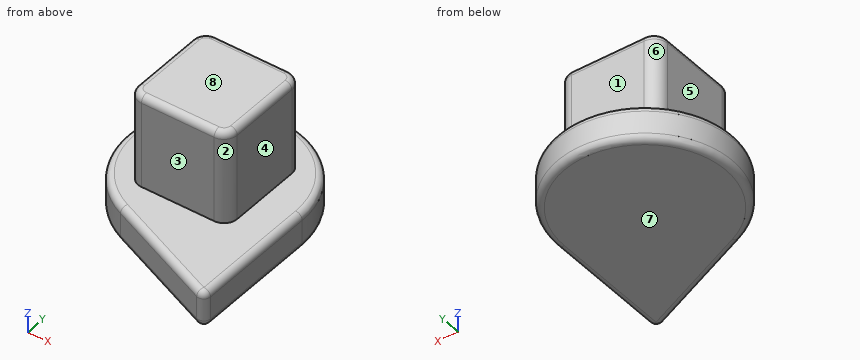
Autodesk Inventor part; units mm, degrees
ref_plane "YZ Plane" through (0, 0, 0) normal (1, 0, 0) x (0, 1, 0)
ref_plane "XZ Plane" through (0, 0, 0) normal (0, 1, 0) x (-1, 0, 0)
ref_plane "XY Plane" through (0, 0, 0) normal (0, 0, 1) x (1, 0, 0)
ref_plane "Work Plane1" through (0, 0, 0) normal (0, 0, 1) x (1, 0, 0)
sketch "Sketch1" plane through (0, 0, 0) normal (0, 0, 1) x (1, 0, 0)
  line L0 (57, -9.5) -> (57, -71.5)
  line L1 (71, -71.5) -> (71, -9.5)
  line L2 (71, -40.5) -> (57, -40.5) construction
  circle A0 centre (64, -40.5) radius 7 construction
  circle A1 centre (64, -40.5) radius 6.6
  line L3 (70.6, -40.5) -> (70.6, -50.5)
  line L4 (70.6, -50.5) -> (61.4052, -46.5685)
  point P0 (0, 0)
  dimension "d0" = 0.4
  dimension "d1" = 10
extrude "Extrusion1" add sketch "Sketch1" along normal blind 2.7
sketch "Sketch2" plane through (0, 0, 2.7) normal (0, 0, 1) x (1, 0, 0)
  line L0 (61.4052, -46.5685) -> (70.6, -50.5)
  line L1 (70.6, -50.5) -> (70.6, -40.5)
  arc A0 (70.6, -40.5) -> (61.4052, -46.5685) centre (64, -40.5) ccw
  line L2 (58.5, -71.5) -> (58.5, -11) construction
  line L3 (69.5, -11) -> (69.5, -71.5) construction
  circle A1 centre (64, -40.5) radius 5.5 construction
  line L4 (60.2523, -36.7523) -> (67.7477, -36.7523)
  line L5 (67.7477, -36.7523) -> (67.7477, -44.2477)
  line L6 (67.7477, -44.2477) -> (60.2523, -44.2477)
  line L7 (60.2523, -44.2477) -> (60.2523, -36.7523)
  line L8 (60.0396, -36.6836) -> (67.9604, -44.3164) construction
  line L9 (67.7477, -36.7523) -> (60.2523, -44.2477) construction
  circle A2 centre (64, -40.5) radius 5.3
  point P0 (0, 0)
  dimension "d11" = 7.4953
  dimension "d12" = 7.4953
  dimension "d14" = 0.2
extrude "Extrusion2" add sketch "Sketch2" along normal blind 7 contours L4 L5 L6 L7
fillet "Fillet1" radius 1 4 edges at (60.2523, -44.2477, 6.2) (60.2523, -36.7523, 6.2) (67.7477, -36.7523, 6.2) (67.7477, -44.2477, 6.2)
fillet "Fillet2" radius 0.5 8 edges at (67.4548, -43.9548, 9.7) (67.7477, -40.5, 9.7) (67.4548, -37.0452, 9.7) (64, -36.7523, 9.7) (60.5452, -37.0452, 9.7) (60.2523, -40.5, 9.7) (60.5452, -43.9548, 9.7) (64, -44.2477, 9.7)
fillet "Fillet3" radius 0.5 7 edges at (60.3644, -34.9916, 2.7) (70.6, -45.5, 2.7) (66.0026, -48.5343, 2.7) (60.3644, -34.9916, 0) (70.6, -45.5, 0) (66.0026, -48.5343, 0) (70.6, -50.5, 1.35)
equation "\"d12\" = d11"
properties part number "Arm"
Source: CAD feature listing. Evaluate the final solid. Frame: model axes, mm. Face numbers are marked on the shaded views. A direction names the side the tool comes from. Give positions to 0.01 mm unless a question says otherwise; leave off trailing zeros. Write each loop counter-clockwise with the first axis right and the second up, starting at its lowest first coordinate (ties: lowest second). Pieces come first, ordered by that corner, then holes. Notation, with made-up numbers: (24.5, 38.25) - (67.5, 38.25) arc R21 cw to (67.5, 62.25) - close; hole circle Ø8 at (-39, -19). An arc over 180 degrees is marked (long way). Write item = value, one per line. Start each with the question number.
Q1. Material intervals for probe 1 along Z at (x, y) = (59.75, -37.25); probe 2 along Y at (x, z) = (62.75, 4); probe 3 along X at (y, z) = (-43.25, 6.5), sorted ascending.
Q2. Reachability of the marked faces 1, 2, 3, 4 and 5 from +Z, -Z, +X, -X, +Y, -Y: full face, straight path, thin tool, end or side. Return the list, or none.
Q3. Pin query (flat end, axial travel): pin 1 Ø1.6 at (y, z) = (-41.5, 7.5) entering from -X; pin 2 Ø4 at (y, z) = (-42.5, 6.5) entering from +X; pin 3 Ø1.6 at (x, z) = (64, 5) entering from +Y. Return the tip coordinate at first contact, or that it passes through.
Q4. Cut plane A-A, the plane z = 9. Return loops of the section in (x, y), then the cut area to 3 significant figures.
Q5. Cut plane C-C, the plane z = 2.5. Return loops of the section in (x, y).
Q6. Draft query along Z for the marked faces 6, 7 and 8. Return one class per face: +Z half, -Z half, draft (parallel to the pull), parting line (faces both ways), or undercut.
Q7. Cut plane B-B, the plane z = 1. Return loops of the section in (x, y), then the cut area to 3 significant figures.
Computed values:
q1.probe_1 = 0 to 2.7
q1.probe_2 = -44.25 to -36.75
q1.probe_3 = 60.25 to 67.75
q2.face_1 = +Z, +X, -X, +Y
q2.face_2 = +Z, +X, -Y
q2.face_3 = +Z, +X, -X, -Y
q2.face_4 = +Z, +X, +Y, -Y
q2.face_5 = +Z, -X, +Y, -Y
q3.pin_1 = 60.25
q3.pin_2 = 67.75
q3.pin_3 = -36.75
q4.outline = (60.25, -43.25) arc R1 ccw to (61.25, -44.25) - (66.75, -44.25) arc R1 ccw to (67.75, -43.25) - (67.75, -37.75) arc R1 ccw to (66.75, -36.75) - (61.25, -36.75) arc R1 ccw to (60.25, -37.75) - close
q4.area = 55.3 mm²
q5.outline = (61.44, -46.48) - (69.94, -50.11) arc R0.4 ccw to (70.5, -49.74) - (70.5, -40.5) arc R6.5 ccw (long way) to start
q6.face_6 = draft
q6.face_7 = -Z half
q6.face_8 = +Z half
q7.outline = (61.41, -46.57) - (69.9, -50.2) arc R0.5 ccw to (70.6, -49.74) - (70.6, -40.5) arc R6.6 ccw (long way) to start
q7.area = 160 mm²
